```python
from build123d import *

# Parameters (mm, degrees)
SKETCH_1_W          = 56
SKETCH_1_H          = 30
EXTRUDE_1_DEPTH     = 12
CUT_EXTRUDE_1_DEPTH = 60.203040462
SKETCH_3_W          = 24
SKETCH_3_H          = 4
CUT_EXTRUDE_2_DEPTH = 43.755116653
EXTRUDE_2_DEPTH     = 8
EXTRUDE_3_DEPTH     = 4


with BuildPart() as part:
    # 草图1 → 凸台-拉伸1 (new body)
    with BuildSketch(Plane(origin=(0, 0, 0), x_dir=(1, 0, 0), z_dir=(0, 1, 0))):
        Rectangle(SKETCH_1_W, SKETCH_1_H)
    extrude(amount=EXTRUDE_1_DEPTH)

    # 草图2 → 切除-拉伸1 (cut, through all)
    with BuildSketch(Plane.ZY.offset(28)):
        Polygon((-6, 0), (-8.886751346, 5), (8.886751346, 5), (6, 0), align=None)
    extrude(amount=-CUT_EXTRUDE_1_DEPTH, mode=Mode.SUBTRACT)

    # 草图3 → 切除-拉伸2 (cut, through all)
    with BuildSketch(Plane.XY.offset(15)):
        with Locations((16, 10)):
            Rectangle(SKETCH_3_W, SKETCH_3_H)
    extrude(amount=-CUT_EXTRUDE_2_DEPTH, mode=Mode.SUBTRACT)

    # 草图4 → 凸台-拉伸2 (add)
    # profile 1 of 2: a face of its own
    with BuildSketch(Plane(origin=(0, 0, -15), x_dir=(-1, 0, 0), z_dir=(0, 0, -1))):
        with BuildLine():
            ThreePointArc((-12.466636051, 32.468013743), (-6.345975777, 28.127398986), (-4, 21))
            Line((-4, 21), (-4, 12))
            Line((-4, 12), (28, 12))
            Line((28, 12), (28, 20))
            Line((28, 20), (-12.466636051, 32.468013743))
        make_face()
    # profile 2 of 2: a face of its own
    with BuildSketch(Plane(origin=(0, 0, -15), x_dir=(-1, 0, 0), z_dir=(0, 0, -1))):
        with BuildLine():
            Line((-4, 12), (-4, 21))
            ThreePointArc((-4, 21), (-6.345975777, 28.127398986), (-12.466636051, 32.468013743))
            ThreePointArc((-12.466636051, 32.468013743), (-23.127398986, 30.654024223), (-28, 21))
            Line((-28, 21), (-28, 8))
            Line((-28, 8), (-4, 8))
            Line((-4, 8), (-4, 12))
        make_face()
        with BuildLine():
            ThreePointArc((-10, 16), (-16, 10), (-22, 16))
            Line((-22, 16), (-22, 21))
            ThreePointArc((-22, 21), (-16, 27), (-10, 21))
            Line((-10, 21), (-10, 16))
        make_face(mode=Mode.SUBTRACT)
    extrude(amount=-EXTRUDE_2_DEPTH)

    # 草图5 → 凸台-拉伸3 (add)
    with BuildSketch(Plane.XY.offset(-7)):
        with BuildLine():
            Line((28, 8), (28, 21))
            ThreePointArc((28, 21), (23.127398986, 30.654024223), (12.466636051, 32.468013743))
            Line((12.466636051, 32.468013743), (4, 29.859392297))
            Line((4, 29.859392297), (4, 12))
            Line((4, 12), (4, 8))
            Line((4, 8), (28, 8))
        make_face()
        with BuildLine():
            Line((22, 21), (22, 16))
            ThreePointArc((22, 16), (16, 10), (10, 16))
            Line((10, 16), (10, 21))
            ThreePointArc((10, 21), (16, 27), (22, 21))
        make_face(mode=Mode.SUBTRACT)
    extrude(amount=EXTRUDE_3_DEPTH)


solid = part.part
```
The model under review builds one solid part; all positions refer to its coordinate system, in mm. A direction names the side the tool comes from. Coordinates: 2 decimals unless noted, no trailing zeros. Write each loop counter-clockwise with the first axis right and the second up, starting at its lowest first coordinate (ties: lowest second). Pieces come first, ordered by that corner, then holes.
1) To check wall thickness, follow probe 1 along X at (y, z) = (19, -10.25); probe 2 along X at (y, z) = (20, -5.75); probe 3 along Y at (x, z) = (-7, 10). State the ranges of each line that lie inside material, in increasing order.
2) We need section C-C on z = -13. State the section outline as (x, y) points, then the cut area to 3 significant figures.
3) We need section A-A on y = 17.5. State the section outline as (x, z) points.
4) Clearance check with flat-ended pins moving along their axes: pin 1 Ø7 at (x, y) = (19, 23) entering from +Z; pin 2 Ø9 at (x, y) = (-13, 18) entering from +Z; pin 3 Ø4.5 at (y, z) = (10.5, 7) entering from +X. State where each tip first meets the part, or that it passes through.
5) The part is to be moulded in two halves that separate along Z. For faces 1 (the face through (23.25, 30.56, -9.08)), 2 (the face through (0, 5, 0)), 3 (the face through (0, 13, -15)), say which applies: pulls with the +Z half, pulls with the -Z half, needs draft (parallel to the pull), parting line crosses it, or undercut.
6) We need section B-B on x = 16. State the section outline as (y, z) points.
7) We need section D-D on x = -3. State the section outline as (y, z) points.
8) Machinability: for faces 4 (the face through (4, 10, 6)), 5 (the face through (0, 0, 10)), 6 (the face through (-0.392, 2.465, -7.423)), 7 (the face through (4, 21, -5)), 8 (the face through (10, 18, -9)), which of the approach directions +Z, -Z, +X, -X, +Y, -Y give a long, thin tool a straight path to every point of the face, cutting with its end or side? Answer none if there is none.
Answer list:
1. probe 1: x = -28 to 10, 22 to 28
1. probe 2: x = 4 to 10, 22 to 28
1. probe 3: y = 0 to 12
2. outline: (-28, 0) - (28, 0) - (28, 21) arc R12 ccw to (12.47, 32.47) - (-28, 20) - close; hole (10, 16) arc R6 ccw to (22, 16) - (22, 21) arc R6 ccw to (10, 21) - close
2. area: 1,370 mm2
3. outline: (-28, -15) - (10, -15) - (10, -3) - (4, -3) - (4, -7) - (-28, -7) - close; (22, -15) - (28, -15) - (28, -3) - (22, -3) - close
4. pin 1: stops at z = -3
4. pin 2: stops at z = -7
4. pin 3: stops at x = 4
5. face 1: needs draft
5. face 2: undercut
5. face 3: pulls with the -Z half
6. outline: (0, -15) - (10, -15) - (10, -3) - (8, -3) - (8, 15) - (0, 15) - (0, 6) - (5, 8.89) - (5, -8.89) - (0, -6) - close; (27, -15) - (33, -15) - (33, -3) - (27, -3) - close
7. outline: (0, -15) - (27.7, -15) - (27.7, -7) - (12, -7) - (12, 15) - (0, 15) - (0, 6) - (5, 8.89) - (5, -8.89) - (0, -6) - close
8. face 4: +Z, +X, +Y
8. face 5: +Z, -Z, +X, -X, -Y
8. face 6: +X, -X
8. face 7: +Z, -X, +Y
8. face 8: +Z, -Z
